Geometry: final body of the model. Coordinates: model frame, mm. Face numbers are marked on the shaded views. A direction names the side the tool comes from. Coordinates: 2 decimals unless noted, no trailing zeros. Write each loop counter-clockwise with the first axis right and the second up, starting at its lowest first coordinate (ties: lowest second). Pieces come first, ordered by that corner, then holes. Notation, with made-up numbers: M -24,11.5 L 8,11.5 A20 ccw 8,20.5 Z; hole C 79.5,19.5 d1. An arc over 180 degrees is marked long. Write item = value, one per line. Start each with the question number.
Item 1: First-contact query: pin 1 Ø10 at (x, y) = (12.5, 14) entering from -Z; pin 2 Ø3.5 at (x, y) = (15, 15) entering from +Z; pin 3 Ø4.5 at (x, z) = (20, -1) entering from +Y; pin 4 Ø10 at (y, z) = (11, 7) entering from +X. Flat tips, straight axial feed; report the tip coordinate or a pass-through.
Item 2: Pull-direction query (X, two-part tool) for the marked faces 1, 2 and 3; classes: +X half, -X half, draft (parallel to the pull), parting line (faces both ways), or undercut.
Item 3: Section B-B on z = 5.75. Output: boundary loops of the cut face in (x, y), plus the area to 3 significant figures.
Item 4: Section C-C on x = 15. Output: boundary loops of the cut face in (y, z), plus the area to 3 significant figures.
Item 5: Section A-A on y = 30. Output: boundary loops of the cut face in (x, z).
Item 6: Section D-D on y = 15. Output: boundary loops of the cut face in (x, z).
Item 7: Reachability of the marked faces 4, 5, 6, 7 and 8 from +Z, -Z, +X, -X, +Y, -Y: full face, straight path, thin tool, end or side. Return the list, or none.
Item 8: Ray query, L1, parallel to Y at x = 15, z = 1; L2, parallel to Y at x = 15, z = 8.1; L3, parallel to Y at x = 24.5, z = 1.25. Return the intervals inside material, ascending. Write a range as [from, to].
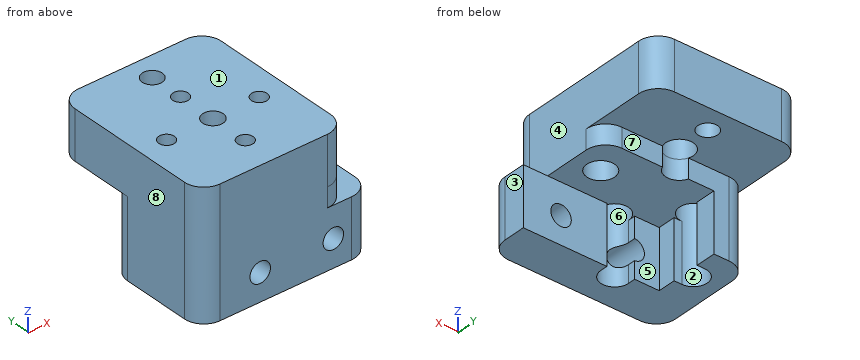
from build123d import *

# Parameters (mm, degrees)
SKETCH1_W           = 30
SKETCH1_H           = 35
SKETCH1_R           = 2.05
SKETCH1_R_2         = 2.1
SKETCH1_R_3         = 1.6
BOSS_EXTRUDE1_DEPTH = 10
SKETCH2_R           = 2.85
CUT_EXTRUDE1_DEPTH  = 5
FILLET1_R           = 4
BOSS_EXTRUDE2_START = -4
SKETCH6_R           = 2.85
BOSS_EXTRUDE2_DEPTH = 4
BOSS_EXTRUDE3_START = 12
BOSS_EXTRUDE3_DEPTH = 12
SKETCH8_R           = 2.1
CUT_EXTRUDE4_DEPTH  = 53.019227215


with BuildPart() as part:
    # Sketch1 → Boss-Extrude1 (new body)
    with BuildSketch(Plane.XY):
        with Locations((15, 17.5)):
            Rectangle(SKETCH1_W, SKETCH1_H)
        with Locations((15, 30)):
            Circle(SKETCH1_R, mode=Mode.SUBTRACT)
        with Locations((15, 15)):
            Circle(SKETCH1_R_2, mode=Mode.SUBTRACT)
        with Locations((5.5, 15)):
            Circle(SKETCH1_R_3, mode=Mode.SUBTRACT)
        with Locations((24.5, 15)):
            Circle(SKETCH1_R_3, mode=Mode.SUBTRACT)
        with Locations((15, 7)):
            Circle(SKETCH1_R_3, mode=Mode.SUBTRACT)
        with Locations((15, 23)):
            Circle(SKETCH1_R_3, mode=Mode.SUBTRACT)
    extrude(amount=BOSS_EXTRUDE1_DEPTH)

    # Sketch2 → Cut-Extrude1 (cut)
    with BuildSketch(Plane(origin=(0, 0, 0), x_dir=(-1, 0, 0), z_dir=(0, 0, -1))):
        with Locations((-15, 7)):
            Circle(SKETCH2_R)
        with Locations((-24.5, 15)):
            Circle(SKETCH2_R)
        with Locations((-15, 23)):
            Circle(SKETCH2_R)
        with Locations((-5.5, 15)):
            Circle(SKETCH2_R)
    extrude(amount=-CUT_EXTRUDE1_DEPTH, mode=Mode.SUBTRACT)

    # Fillet1
    fillet1_edges = [part.edges().sort_by_distance(p)[0] for p in [
        (0, 35, 5),
        (30, 35, 5),
        (30, 0, 5),
        (0, 0, 5),
    ]]
    fillet(fillet1_edges, radius=FILLET1_R)

    # Sketch6 → Boss-Extrude2 (add)
    with BuildSketch(Plane.XY.offset(BOSS_EXTRUDE2_START)):
        with BuildLine():
            Line((26, 22), (17.668801229, 22))
            ThreePointArc((17.668801229, 22), (15, 20.15), (12.331198771, 22))
            Line((12.331198771, 22), (4, 22))
            ThreePointArc((4, 22), (1.171572875, 20.828427125), (0, 18))
            Line((0, 18), (0, 4))
            ThreePointArc((0, 4), (1.171572875, 1.171572875), (4, 0))
            Line((4, 0), (26, 0))
            ThreePointArc((26, 0), (28.828427125, 1.171572875), (30, 4))
            Line((30, 4), (30, 18))
            ThreePointArc((30, 18), (28.828427125, 20.828427125), (26, 22))
        make_face()
        with Locations(Location((5.5, 15, 0), (0, 0, 180))):
            Circle(SKETCH6_R, mode=Mode.SUBTRACT)
        with Locations(Location((15, 7, 0), (0, 0, 180))):
            Circle(SKETCH6_R, mode=Mode.SUBTRACT)
        with Locations(Location((24.5, 15, 0), (0, 0, 180))):
            Circle(SKETCH6_R, mode=Mode.SUBTRACT)
    extrude(amount=BOSS_EXTRUDE2_DEPTH)

    # Sketch7 → Boss-Extrude3 (add)
    with BuildSketch(Plane(origin=(0, 0, -4), x_dir=(-1, 0, 0), z_dir=(0, 0, -1)).offset(BOSS_EXTRUDE3_START)):
        with BuildLine():
            Line((-7.1, 22), (-7.1, 17.85))
            Line((-7.1, 17.85), (-5.5, 17.85))
            ThreePointArc((-5.5, 17.85), (-2.65, 15), (-5.5, 12.15))
            Line((-5.5, 12.15), (-7.1, 12.15))
            Line((-7.1, 12.15), (-7.1, 8.5))
            Line((-7.1, 8.5), (-12.15, 8.5))
            Line((-12.15, 8.5), (-12.15, 7))
            ThreePointArc((-12.15, 7), (-15, 4.15), (-17.85, 7))
            Line((-17.85, 7), (-17.85, 8.5))
            Line((-17.85, 8.5), (-30, 8.5))
            Line((-30, 8.5), (-35, 8.5))
            Line((-35, 8.5), (-35, 4))
            ThreePointArc((-35, 4), (-33.828427125, 1.171572875), (-31, 0))
            Line((-31, 0), (-26, 0))
            Line((-26, 0), (-4, 0))
            ThreePointArc((-4, 0), (-1.171572875, 1.171572875), (0, 4))
            Line((0, 4), (0, 18))
            ThreePointArc((0, 18), (-1.171572875, 20.828427125), (-4, 22))
            Line((-4, 22), (-7.1, 22))
        make_face()
    extrude(amount=-BOSS_EXTRUDE3_DEPTH)

    # Sketch8 → Cut-Extrude4 (cut, through all)
    with BuildSketch(Plane.XZ):
        with Locations(Location((12.249401243, -10.35, 0), (0, 0, 270))):
            Circle(SKETCH8_R)
        with Locations(Location((27.249401243, -10.35, 0), (0, 0, 270))):
            Circle(SKETCH8_R)
    extrude(amount=-CUT_EXTRUDE4_DEPTH, mode=Mode.SUBTRACT)


solid = part.part
Responses:
q1.pin_1 = -4
q1.pin_2 = 0
q1.pin_3 = 35
q1.pin_4 = 30
q2.face_1 = draft
q2.face_2 = undercut
q2.face_3 = +X half
q3.outline = M 0,4 A4 ccw 4,0 L 26,0 A4 ccw 30,4 L 30,31 A4 ccw 26,35 L 4,35 A4 ccw 0,31 Z; hole C 5.5,15 d3.2; hole C 15,15 d4.2; hole C 15,30 d4.1; hole C 15,7 d3.2; hole C 15,23 d3.2; hole C 24.5,15 d3.2
q3.area = 977 mm²
q4.outline = M 0,-16 L 4.15,-16 L 4.15,5 L 5.4,5 L 5.4,10 L 0,10 Z; M 8.6,5 L 9.85,5 L 9.85,-4 L 20.15,-4 L 20.15,5 L 21.4,5 L 21.4,10 L 17.1,10 L 17.1,0 L 12.9,0 L 12.9,10 L 8.6,10 Z; M 24.6,5 L 25.85,5 L 25.85,0 L 27.95,0 L 27.95,10 L 24.6,10 Z; M 32.05,0 L 35,0 L 35,10 L 32.05,10 Z
q4.area = 286 mm²
q5.outline = M 0,0 L 12.95,0 L 12.95,10 L 0,10 Z; M 17.05,0 L 30,0 L 30,10 L 17.05,10 Z
q6.outline = M 0,-16 L 2.65,-16 L 2.65,5 L 3.9,5 L 3.9,10 L 0,10 Z; M 7.1,5 L 8.35,5 L 8.35,-4 L 21.65,-4 L 21.65,5 L 22.9,5 L 22.9,10 L 17.1,10 L 17.1,0 L 12.9,0 L 12.9,10 L 7.1,10 Z; M 26.1,5 L 27.35,5 L 27.35,-4 L 30,-4 L 30,10 L 26.1,10 Z
q7.face_4 = +Z, +X, +Y, -Y
q7.face_5 = -Z, +X, +Y
q7.face_6 = -Z
q7.face_7 = -Z, +X, -X, +Y
q7.face_8 = +Z, -Z, -X, +Y, -Y
q8.L1 = [0, 4.15], [9.85, 12.9], [17.1, 20.15], [25.85, 27.95], [32.05, 35]
q8.L2 = [0, 5.4], [8.6, 12.9], [17.1, 21.4], [24.6, 27.95], [32.05, 35]
q8.L3 = [0, 12.15], [17.85, 35]
